```python
from build123d import *

# Parameters (mm, degrees)
SKETCH2_R           = 7.9375
BOSS_EXTRUDE1_DEPTH = 18.415
CHAMFER1_SIZE       = 1.27
CUT_EXTRUDE2_DEPTH  = 15.24
SKETCH5_R           = 3.81
CUT_EXTRUDE3_DEPTH  = 3.175


with BuildPart() as part:
    # Sketch2 → Boss-Extrude1 (new body)
    with BuildSketch(Plane(origin=(0, 0, 0), x_dir=(0, 0, -1), z_dir=(1, 0, 0))):
        Circle(SKETCH2_R)
    extrude(amount=BOSS_EXTRUDE1_DEPTH)

    # Chamfer1
    chamfer1_edges = [part.edges().sort_by_distance(p)[0] for p in [
        (0, 0, 7.9375),
        (18.415, 0, 7.9375),
    ]]
    chamfer(chamfer1_edges, length=CHAMFER1_SIZE)

    # Sketch4 → Cut-Extrude2 (cut)
    with BuildSketch(Plane.ZY):
        with BuildLine():
            Line((-2.851142929, 1.397), (2.851142929, 1.397))
            ThreePointArc((2.851142929, 1.397), (0, -3.175), (-2.851142929, 1.397))
        make_face()
    extrude(amount=-CUT_EXTRUDE2_DEPTH, mode=Mode.SUBTRACT)

    # Sketch5 → Cut-Extrude3 (cut)
    with BuildSketch(Plane.ZY):
        Circle(SKETCH5_R)
    extrude(amount=-CUT_EXTRUDE3_DEPTH, mode=Mode.SUBTRACT)


solid = part.part
```
Could you check a few things on this model? Use its own coordinates, in mm. A direction names the side the tool comes from. Round coordinates to 2 decimals unless told otherwise and drop trailing zeros. Loops run counter-clockwise (first coordinate to the right, second up) from the corner with the lowest first, then second, coordinate; pieces in that order, holes last. Notation, with made-up numbers: (59.25, -0.75) - (105.25, -0.75) arc R23 ccw to (105.25, 36.25) - close; hole circle Ø10 at (58.25, 72). An arc over 180 degrees is marked (long way). Answer in a Markdown table with one row per item. Add a question column.
(1) If we section it at B-B (z = 0): Please give me the cut outline in (x, y) (1 decimal), plus the area to 3 significant figures.
(2) I'm going to push flat-ended pins straight in: pin 1 (2 mm diameter, centred on x = 9.5, z = -3, fed in from -Y); pin 2 (2.5 mm diameter, centred on y = 0, z = -1, fed in from -X); pin 3 (1 mm diameter, centred on x = 5.5, z = -2, fed in from -Y). Where does each tip first touch, or does it pass through?
(3) I need wall thicknesses on line 1 along Z through (x, y) = (10.75, -2); line 2 along Y through (x, z) = (11, 2); line 3 along Z through (x, y) = (3.75, -0.5). Which ranges of each line are inside material? Lowest first, please.
(4) If we section it at A-A (y = 0): Please give me the cut outline in (x, z) (1 decimal), plus the area to 3 significant figures.
(5) For faces 5 (the face through (18.415, 0, 0)), 6 (the face through (3.175, 2, 0)), which set-ups out of +Z, -Z, +X, -X, +Y, -Y let a thin tool reach every point of the face, with its end or its side?
(6) If we mould it in two halves opening along Z, with no side actions, what happens to faces 1 (the face through (9.1, -7.75, 1.72)), 2 (the face through (0, -3, -3)), 3 (the face through (9, 1.397, 0)), 4 (the face through (1.57, -3.72, -0.83))? For each: pulls with the +Z half, pulls with the -Z half, needs draft (parallel to the pull), parting line crosses it, or undercut.
Model answer:
| question | item | result |
|---|---|---|
| 1 | outline | (0, -6.7) - (1.3, -7.9) - (17.1, -7.9) - (18.4, -6.7) - (18.4, 6.7) - (17.1, 7.9) - (1.3, 7.9) - (0, 6.7) - (0, 3.8) - (3.2, 3.8) - (3.2, 1.4) - (15.2, 1.4) - (15.2, -3.2) - (3.2, -3.2) - (3.2, -3.8) - (0, -3.8) - close |
| 1 | area | 210 mm² |
| 2 | pin 1 | stops at y = -7.68 |
| 2 | pin 2 | stops at x = 15.24 |
| 2 | pin 3 | stops at y = -7.79 |
| 3 | line 1 | z = -7.68 to -2.47, 2.47 to 7.68 |
| 3 | line 2 | y = -7.68 to -2.47, 1.4 to 7.68 |
| 3 | line 3 | z = -7.92 to -3.14, 3.14 to 7.92 |
| 4 | outline | (0, -6.7) - (1.3, -7.9) - (17.1, -7.9) - (18.4, -6.7) - (18.4, 6.7) - (17.1, 7.9) - (1.3, 7.9) - (0, 6.7) - (0, 3.8) - (3.2, 3.8) - (3.2, 3.2) - (15.2, 3.2) - (15.2, -3.2) - (3.2, -3.2) - (3.2, -3.8) - (0, -3.8) - close |
| 4 | area | 188 mm² |
| 5 | face 5 | +Z, -Z, +X, +Y, -Y |
| 5 | face 6 | -X |
| 6 | face 1 | parting line crosses it |
| 6 | face 2 | needs draft |
| 6 | face 3 | undercut |
| 6 | face 4 | undercut |
